Design review of the part built by this model. Coordinates are the model's own, in mm. Face numbers are marked on the shaded views. A direction names the side the tool comes from. Coordinates: 2 decimals unless noted, no trailing zeros. Loops run counter-clockwise (first coordinate to the right, second up) from the corner with the lowest first, then second, coordinate; pieces in that order, holes last. Notation, with made-up numbers: (3, 35.25) -> (49, 35.25) arc R25 ccw to (49, 67.25) -> close; hole circle Ø10 at (49.25, 28.25). An arc over 180 degrees is marked (long way). Use a Markdown table: item, result. Add a question column.
Q1. Draft analysis for pull direction Z (two halves, no side actions). For the marked faces 1, 2 and 3, state which applies: pulls with the +Z half, pulls with the -Z half, needs draft (parallel to the pull), parting line crosses it, or undercut.
Q2. Take a section at A-A on x = 0. Write out the cut boundary in (y, z), plus the area to 3 significant figures.
Q3. Take a section at C-C on y = -11.5. Write out the cut boundary in (x, z), plus the area to 3 significant figures.
Q4. Take a section at B-B on z = -13.5. Write out the cut boundary in (x, y).
Q5. For the marked faces 4, 5, 6 and 7, list the 3-axis set-ups (+Z, -Z, +X, -X, +Y, -Y) from which the entire face can be reached by the end or side of a thin tool; tool diameter is ignored.
Q6. For probe 1 along X at (y, z) = (0.4, 0); probe 2 along X at (y, z) = (-43, -14); probe 3 along Y at (x, z) = (15, 2.5), list the stretches that pass through material, from the lowest coordinate up.
Q7. Clearance check with flat-ended pins moving along their axes: pin 1 Ø7 at (x, y) = (0, -45.59) entering from -Z; pin 2 Ø1.5 at (x, y) = (18, -12.5) entering from +Z; pin 3 Ø1.5 at (x, z) = (-11, 8) entering from +Y; pin 4 Ø5 at (x, y) = (-5, -46) entering from -Z. State where each tip first meets the part, or that it passes through.
Q8. Take a section at D-D on z = 3. Write out the cut boundary in (x, y), plus the area to 3 significant figures.
from build123d import *

# Parameters (mm, degrees)
SKETCH1_R           = 32.5
SKETCH1_R_2         = 30
BOSS_EXTRUDE3_DEPTH = 10
BOSS_EXTRUDE4_DEPTH = 63.5872
BOSS_EXTRUDE5_DEPTH = 10
SKETCH2_R           = 6
CUT_EXTRUDE1_DEPTH  = 45
SKETCH3_R           = 8
SKETCH3_R_2         = 6
BOSS_EXTRUDE6_DEPTH = 2


with BuildPart() as part:
    # Sketch1 → Boss-Extrude3 (new body)
    with BuildSketch(Plane(origin=(0, 0, 0), x_dir=(1, 0, 0), z_dir=(0, 1, 0))):
        with Locations(Location((0, 0, 0), (0, 0, 270))):
            Circle(SKETCH1_R)
        with Locations(Location((0, 0, 0), (0, 0, 270))):
            Circle(SKETCH1_R_2, mode=Mode.SUBTRACT)
    extrude(amount=-BOSS_EXTRUDE3_DEPTH)

    # Sketch1_3 → Boss-Extrude4 (add)
    with BuildSketch(Plane(origin=(0, 0, 0), x_dir=(1, 0, 0), z_dir=(0, 1, 0))):
        with BuildLine():
            Line((-30, 0), (30, 0))
            ThreePointArc((30, 0), (0, 30), (-30, 0))
        make_face()
    extrude(amount=-BOSS_EXTRUDE4_DEPTH)

    # Sketch1_4 → Boss-Extrude5 (add)
    with BuildSketch(Plane(origin=(0, 0, 0), x_dir=(1, 0, 0), z_dir=(0, 1, 0))):
        with BuildLine():
            ThreePointArc((-30, 0), (0, -30), (30, 0))
            Line((30, 0), (-30, 0))
        make_face()
        with BuildLine():
            Line((-30, 0), (30, 0))
            ThreePointArc((30, 0), (0, 30), (-30, 0))
        make_face()
    extrude(amount=-BOSS_EXTRUDE5_DEPTH)

    # Sketch2 → Cut-Extrude1 (cut)
    with BuildSketch(Plane.XY):
        with Locations((0, -45.5872)):
            Circle(SKETCH2_R)
    extrude(amount=-CUT_EXTRUDE1_DEPTH, mode=Mode.SUBTRACT)

    # Sketch3 → Boss-Extrude6 (add)
    with BuildSketch(Plane(origin=(0, 0, 0), x_dir=(1, 0, 0), z_dir=(0, 1, 0))):
        with Locations(Location((0, 0, 0), (0, 0, 270))):
            Circle(SKETCH3_R)
        with Locations(Location((0, 0, 0), (0, 0, 270))):
            Circle(SKETCH3_R_2, mode=Mode.SUBTRACT)
    extrude(amount=BOSS_EXTRUDE6_DEPTH)


solid = part.part
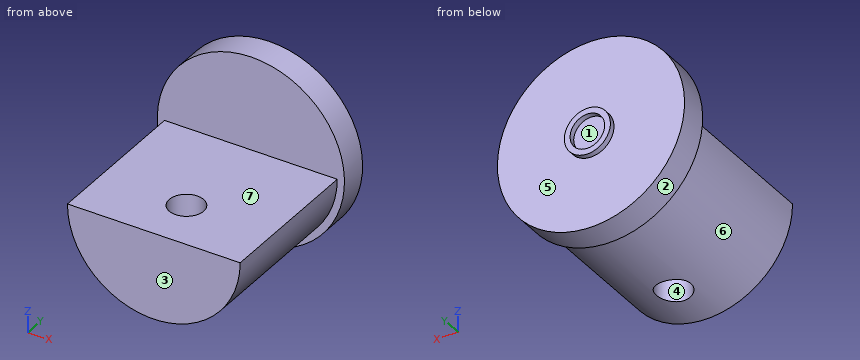
Answer list:
| question | item | result |
|---|---|---|
| 1 | face 1 | undercut |
| 1 | face 2 | parting line crosses it |
| 1 | face 3 | needs draft |
| 2 | outline | (-63.59, -30) -> (-51.59, -30) -> (-51.59, 0) -> (-63.59, 0) -> close; (-39.59, -30) -> (-10, -30) -> (-10, -32.5) -> (0, -32.5) -> (0, -8) -> (2, -8) -> (2, -6) -> (0, -6) -> (0, 6) -> (2, 6) -> (2, 8) -> (0, 8) -> (0, 32.5) -> (-10, 32.5) -> (-10, 0) -> (-39.59, 0) -> close |
| 2 | area | 1,910 mm² |
| 3 | outline | (-30, 0) arc R30 ccw to (30, 0) -> close |
| 3 | area | 1,410 mm² |
| 4 | outline | (-29.56, -10) -> (-26.79, -10) -> (-26.79, -63.59) -> (26.79, -63.59) -> (26.79, -10) -> (29.56, -10) -> (29.56, 0) -> (-29.56, 0) -> close; hole circle Ø12 at (0, -45.59) |
| 5 | face 4 | +Z, -Z |
| 5 | face 5 | +Y |
| 5 | face 6 | -Z, -Y |
| 5 | face 7 | +Z, +X, -X, -Y |
| 6 | probe 1 | -8 to -6, 6 to 8 |
| 6 | probe 2 | -26.53 to -5.41, 5.41 to 26.53 |
| 6 | probe 3 | -10 to 0 |
| 7 | pin 1 | through |
| 7 | pin 2 | z = 0 |
| 7 | pin 3 | y = 0 |
| 7 | pin 4 | z = -29.54 |
| 8 | outline | (-32.36, -10) -> (32.36, -10) -> (32.36, 0) -> (7.42, 0) -> (7.42, 2) -> (5.2, 2) -> (5.2, 0) -> (-5.2, 0) -> (-5.2, 2) -> (-7.42, 2) -> (-7.42, 0) -> (-32.36, 0) -> close |
| 8 | area | 656 mm² |
